```python
from build123d import *
from build123d import SkipClean  # not in build123d's __all__

# Parameters (mm, degrees)
F0_R     = 41.5
F0_R_2   = 36
F1_DEPTH = 35
F0_R_3   = 47.5
F2_DEPTH = 10
F3_DEPTH = 5
F4_R     = 2
F5_SIZE  = 2
F7_DEPTH = 40.1


with BuildPart() as f1:
    # F0 (on Top) → F1 (new body)
    with BuildSketch(Plane.XY):
        Circle(F0_R)
        Circle(F0_R_2, mode=Mode.SUBTRACT)
    extrude(amount=F1_DEPTH)

    # F0 (on Top) → F2 (join)
    with BuildSketch(Plane.XY):
        Circle(F0_R_3)
        Circle(F0_R, mode=Mode.SUBTRACT)
    extrude(amount=F2_DEPTH)

    # F0 (on Top) → F3 (join)
    with BuildSketch(Plane.XY):
        Circle(F0_R_2)
    extrude(amount=F3_DEPTH)

    # F4
    f4_edges = [f1.edges().sort_by_distance(p)[0] for p in [
        (-41.5, 0, 35),
        (-36, 0, 35),
    ]]
    fillet(f4_edges, radius=F4_R)

    # F5
    f5_edges = [f1.edges().sort_by_distance(p)[0] for p in [
        (-47.5, 0, 0),
    ]]
    chamfer(f5_edges, length=F5_SIZE)

    # F6 (on face) → F7 (cut)
    with BuildSketch(Plane.XY):
        with BuildLine():
            ThreePointArc((27.3098579389, -2.5), (19.3917294309, -19.3917294309), (2.5, -27.3098579389))
            Line((2.5, -27.3098579389), (2.5, -35.9130895357))
            ThreePointArc((2.5, -35.9130895357), (25.4558441227, -25.4558441227), (35.9130895357, -2.5))
            Line((35.9130895357, -2.5), (27.3098579389, -2.5))
        make_face()
        with BuildLine():
            Line((-2.5, -35.9130895357), (-2.5, -27.3098579389))
            ThreePointArc((-2.5, -27.3098579389), (-19.3917294309, -19.3917294309), (-27.3098579389, -2.5))
            Line((-27.3098579389, -2.5), (-35.9130895357, -2.5))
            ThreePointArc((-35.9130895357, -2.5), (-25.4558441227, -25.4558441227), (-2.5, -35.9130895357))
        make_face()
        with BuildLine():
            ThreePointArc((-27.3098579389, 2.5), (-19.3917294309, 19.3917294309), (-2.5, 27.3098579389))
            Line((-2.5, 27.3098579389), (-2.5, 35.9130895357))
            ThreePointArc((-2.5, 35.9130895357), (-25.4558441227, 25.4558441227), (-35.9130895357, 2.5))
            Line((-35.9130895357, 2.5), (-27.3098579389, 2.5))
        make_face()
        with BuildLine():
            Line((2.5, 35.9130895357), (2.5, 27.3098579389))
            ThreePointArc((2.5, 27.3098579389), (19.3917294309, 19.3917294309), (27.3098579389, 2.5))
            Line((27.3098579389, 2.5), (35.9130895357, 2.5))
            ThreePointArc((35.9130895357, 2.5), (25.4558441227, 25.4558441227), (2.5, 35.9130895357))
        make_face()
        with BuildLine():
            Line((2.5, 17.8404992818), (2.5, 8.7134999292))
            ThreePointArc((2.5, 8.7134999292), (6.4099563577, 6.4099563577), (8.7134999292, 2.5))
            Line((8.7134999292, 2.5), (17.8404992818, 2.5))
            ThreePointArc((17.8404992818, 2.5), (12.7383950053, 12.7383950053), (2.5, 17.8404992818))
        make_face()
        with BuildLine():
            ThreePointArc((8.7134999292, -2.5), (6.4099563577, -6.4099563577), (2.5, -8.7134999292))
            Line((2.5, -8.7134999292), (2.5, -17.8404992818))
            ThreePointArc((2.5, -17.8404992818), (12.7383950053, -12.7383950053), (17.8404992818, -2.5))
            Line((17.8404992818, -2.5), (8.7134999292, -2.5))
        make_face()
        with BuildLine():
            Line((-2.5, -17.8404992818), (-2.5, -8.7134999292))
            ThreePointArc((-2.5, -8.7134999292), (-6.4099563577, -6.4099563577), (-8.7134999292, -2.5))
            Line((-8.7134999292, -2.5), (-17.8404992818, -2.5))
            ThreePointArc((-17.8404992818, -2.5), (-12.7383950053, -12.7383950053), (-2.5, -17.8404992818))
        make_face()
        with BuildLine():
            ThreePointArc((-8.7134999292, 2.5), (-6.4099563577, 6.4099563577), (-2.5, 8.7134999292))
            Line((-2.5, 8.7134999292), (-2.5, 17.8404992818))
            ThreePointArc((-2.5, 17.8404992818), (-12.7383950053, 12.7383950053), (-17.8404992818, 2.5))
            Line((-17.8404992818, 2.5), (-8.7134999292, 2.5))
        make_face()
    with SkipClean():  # cleaning this boolean's faces spoils the solid; the shape is the same uncleaned
        extrude(amount=F7_DEPTH, mode=Mode.SUBTRACT)


solid = f1.part
```
Geometry check sheet. Reference: the model listing, model coordinates, mm. Round coordinates to 2 decimals unless told otherwise and drop trailing zeros. Order: outer loops, then holes, each group sorted by start corner. A loop starts at its lowest first (then second) coordinate and runs counter-clockwise, first axis right, second up. Notation, with made-up numbers: (39, 36.25) -> (79, 36.25) arc R13 ccw to (79, 54.25) -> close; hole circle Ø11 at (89, -14.5). An arc over 180 degrees is marked (long way). Return JSON: item names as keys, results as strings. Group by question number.
Q1. Section check B-B, the plane z = 20.5. Record the boundary of the cut face in (x, y).
Q2. Release check for a two-part mould opening along Y. For faces 1 (the cylindrical face through (19.2, 19.58, 2.46)), 2 (the flat face through (-1, 1, 0)) record: released by +Y, released by -Y, zero draft, split by the parting line, or undercut.
Q3. Material ranges on probe 1 along X at (y, z) = (15, 4); probe 2 along Y at (x, z) = (-6.5, 3.5); probe 3 along Y at (x, z) = (21, 2), recorded low to high. Write a range as from..to.
Q4. Gauge pin test, flat ends, axial feed: pin 1 (5.5 mm diameter, centred on x = 33, z = 2, fed in from +Y); pin 2 (1 mm diameter, centred on y = 7, z = 11, fed in from -X); pin 3 (1.5 mm diameter, centred on x = -11.5, z = 3.5, fed in from +Y). Record the tip position at first contact, or that the pin passes through.
Q5. Section check A-A, the plane x = 0. Record the boundary of the cut face in (y, z).
Q6. Section check C-C, the plane y = 29. Count the separate pieces of the cut face and the enclosed holes in it, plus the area to 3 significant figures.
Numbers:
{
 "1": {"outline": "circle Ø83 at (0, 0); hole circle Ø72 at (0, 0)"},
 "2": {"face 1": "undercut", "face 2": "zero draft"},
 "3": {"probe 1": "-45.07..-32.73, -22.96..-9.98, -2.5..2.5, 9.98..22.96, 32.73..45.07", "probe 2": "-47.05..-35.41, -26.64..-16.8, -6.32..6.32, 16.8..26.64, 35.41..47.05", "probe 3": "-42.61..-29.24, -17.64..17.64, 29.24..42.61"},
 "4": {"pin 1": "y = 36.62", "pin 2": "x = -40.99", "pin 3": "y = 46.27"},
 "5": {"outline": "(-47.5, 2) -> (-45.5, 0) -> (45.5, 0) -> (47.5, 2) -> (47.5, 10) -> (41.5, 10) -> (41.5, 33) arc R2 ccw to (39.5, 35) -> (38, 35) arc R2 ccw to (36, 33) -> (36, 5) -> (-36, 5) -> (-36, 33) arc R2 ccw to (-38, 35) -> (-39.5, 35) arc R2 ccw to (-41.5, 33) -> (-41.5, 10) -> (-47.5, 10) -> close"},
 "6": {"separate pieces": "3", "enclosed holes": "0", "area": "758 mm^2"}
}
